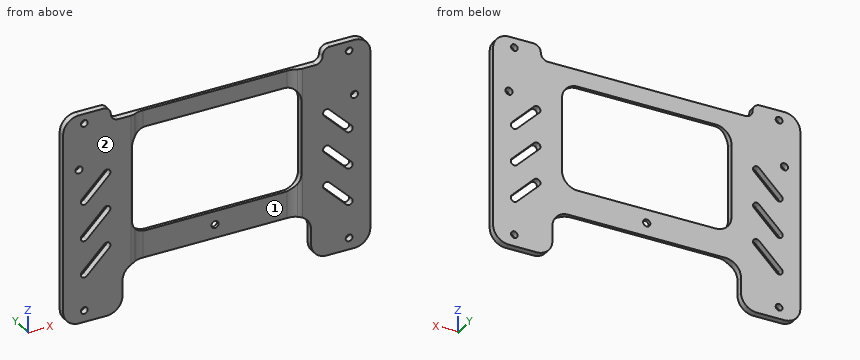
from build123d import *

# Parameters (mm, degrees)
SKETCH_1_R          = 1.7
EXTRUDE_1_DEPTH     = 3
FILLET_1_R          = 7.5
FILLET_2_R          = 3.5
CUT_EXTRUDE_5_DEPTH = 10
CUT_EXTRUDE_6_DEPTH = 10
CUT_EXTRUDE_7_DEPTH = 1.5
FILLET_START        = -35.28
FILLET_3_DEPTH      = 78.28
FILLET_4_R          = 10


with BuildPart() as part:
    # 草图1 → 凸台-拉伸1 (new body)
    with BuildSketch(Plane(origin=(0, 0, 0), x_dir=(1, 0, 0), z_dir=(0, 1, 0))):
        Polygon((-67.5, 50), (-44.5, 50), (-44.5, 27.78), (44.5, 27.78), (44.5, 50), (67.5, 50), (72.5, 50), (72.5, -50), (67.5, -50), (50, -50), (50, -43), (0, -43), (-50, -43), (-50, -50), (-67.5, -50), (-72.5, -50), (-72.5, 50), align=None)
        with Locations(Location((0, 21.39, 0), (0, 0, 270))):
            Circle(SKETCH_1_R, mode=Mode.SUBTRACT)
        with Locations(Location((65, -23.76, 0), (0, 0, 270))):
            Circle(SKETCH_1_R, mode=Mode.SUBTRACT)
        with Locations(Location((-65, -23.76, 0), (0, 0, 270))):
            Circle(SKETCH_1_R, mode=Mode.SUBTRACT)
        Polygon((-40, -10), (-40, -35), (40, -35), (40, 15), (-40, 15), align=None, mode=Mode.SUBTRACT)
    extrude(amount=EXTRUDE_1_DEPTH)

    # 圆角1
    fillet_1_edges = [part.edges().sort_by_distance(p)[0] for p in [
        (72.5, 1.5, -50),
        (72.5, 1.5, 50),
        (-72.5, 1.5, 50),
        (-72.5, 1.5, -50),
        (-44.5, 1.5, -50),
        (-44.5, 1.5, -27.78),
        (44.5, 1.5, -27.78),
        (44.5, 1.5, -50),
        (-40, 1.5, -15),
        (-40, 1.5, 35),
        (40, 1.5, 35),
        (40, 1.5, -15),
    ]]
    fillet(fillet_1_edges, radius=FILLET_1_R)

    # 圆角2
    fillet_2_edges = [part.edges().sort_by_distance(p)[0] for p in [
        (50, 1.5, 43),
        (-50, 1.5, 43),
    ]]
    fillet(fillet_2_edges, radius=FILLET_2_R)
    fillet_2_2_edges = [part.edges().sort_by_distance(p)[0] for p in [
        (50, 1.5, 50),
        (-50, 1.5, 50),
    ]]
    fillet(fillet_2_2_edges, radius=FILLET_2_R - 0.0001)  # a hair under: the kernel refuses the full size

    # 草图12 → 切除-拉伸5 (cut)
    with BuildSketch(Plane(origin=(0, 0, 0), x_dir=(-1, 0, 0), z_dir=(0, -1, 0))):
        with BuildLine():
            ThreePointArc((62.47765, -43.808317961), (61.34627915, -44.276947111), (60.87765, -45.408317961))
            Line((60.87765, -45.408317961), (62.47765, -45.408317961))
            Line((62.47765, -45.408317961), (62.47765, -43.808317961))
        make_face()
        with BuildLine():
            Line((62.47765, -45.408317961), (60.87765, -45.408317961))
            ThreePointArc((60.87765, -45.408317961), (62.47765, -47.008317961), (64.07765, -45.408317961))
            ThreePointArc((64.07765, -45.408317961), (63.60902085, -44.276947111), (62.47765, -43.808317961))
            Line((62.47765, -43.808317961), (62.47765, -45.408317961))
        make_face()
        with BuildLine():
            ThreePointArc((-62.47765, -43.808317961), (-63.60902085, -46.539688811), (-60.87765, -45.408317961))
            Line((-60.87765, -45.408317961), (-62.47765, -45.408317961))
            Line((-62.47765, -45.408317961), (-62.47765, -43.808317961))
        make_face()
        with BuildLine():
            Line((-62.47765, -45.408317961), (-60.87765, -45.408317961))
            ThreePointArc((-60.87765, -45.408317961), (-61.34627915, -44.276947111), (-62.47765, -43.808317961))
            Line((-62.47765, -43.808317961), (-62.47765, -45.408317961))
        make_face()
        with BuildLine():
            ThreePointArc((-62.47765, 42.891807039), (-61.34627915, 43.360436189), (-60.87765, 44.491807039))
            Line((-60.87765, 44.491807039), (-62.47765, 44.491807039))
            Line((-62.47765, 44.491807039), (-62.47765, 42.891807039))
        make_face()
        with BuildLine():
            Line((-62.47765, 44.491807039), (-60.87765, 44.491807039))
            ThreePointArc((-60.87765, 44.491807039), (-63.60902085, 45.623177889), (-62.47765, 42.891807039))
            Line((-62.47765, 42.891807039), (-62.47765, 44.491807039))
        make_face()
        with BuildLine():
            ThreePointArc((64.07765, 44.491807039), (62.47765, 46.091807039), (60.87765, 44.491807039))
            Line((60.87765, 44.491807039), (62.47765, 44.491807039))
            Line((62.47765, 44.491807039), (62.47765, 42.891807039))
            ThreePointArc((62.47765, 42.891807039), (63.60902085, 43.360436189), (64.07765, 44.491807039))
        make_face()
        with BuildLine():
            Line((62.47765, 44.491807039), (60.87765, 44.491807039))
            ThreePointArc((60.87765, 44.491807039), (61.34627915, 43.360436189), (62.47765, 42.891807039))
            Line((62.47765, 42.891807039), (62.47765, 44.491807039))
        make_face()
    extrude(amount=-CUT_EXTRUDE_5_DEPTH, mode=Mode.SUBTRACT)

    # 草图13 → 切除-拉伸6 (cut)
    with BuildSketch(Plane(origin=(0, 3, 0), x_dir=(1, 0, 0), z_dir=(0, 1, 0))):
        with BuildLine():
            Line((61.275568472, -6.806111433), (50.668966754, -17.412713151))
            ThreePointArc((50.668966754, -17.412713151), (50.668966754, -19.816876207), (53.07312981, -19.816876207))
            Line((53.07312981, -19.816876207), (63.679731528, -9.210274489))
            ThreePointArc((63.679731528, -9.210274489), (63.679731528, -6.806111433), (61.275568472, -6.806111433))
        make_face()
        with BuildLine():
            Line((-61.275568472, 28.193888567), (-50.668966754, 17.587286849))
            ThreePointArc((-50.668966754, 17.587286849), (-50.668966754, 15.183123793), (-53.07312981, 15.183123793))
            Line((-53.07312981, 15.183123793), (-63.679731528, 25.789725511))
            ThreePointArc((-63.679731528, 25.789725511), (-63.679731528, 28.193888567), (-61.275568472, 28.193888567))
        make_face()
        with BuildLine():
            Line((-63.679731528, 8.289725511), (-53.07312981, -2.316876207))
            ThreePointArc((-53.07312981, -2.316876207), (-50.668966754, -2.316876207), (-50.668966754, 0.087286849))
            Line((-50.668966754, 0.087286849), (-61.275568472, 10.693888567))
            ThreePointArc((-61.275568472, 10.693888567), (-63.679731528, 10.693888567), (-63.679731528, 8.289725511))
        make_face()
        with BuildLine():
            Line((-63.679731528, -9.210274489), (-53.07312981, -19.816876207))
            ThreePointArc((-53.07312981, -19.816876207), (-50.668966754, -19.816876207), (-50.668966754, -17.412713151))
            Line((-50.668966754, -17.412713151), (-61.275568472, -6.806111433))
            ThreePointArc((-61.275568472, -6.806111433), (-63.679731528, -6.806111433), (-63.679731528, -9.210274489))
        make_face()
        with BuildLine():
            Line((61.275568472, 10.693888567), (50.668966754, 0.087286849))
            ThreePointArc((50.668966754, 0.087286849), (50.668966754, -2.316876207), (53.07312981, -2.316876207))
            Line((53.07312981, -2.316876207), (63.679731528, 8.289725511))
            ThreePointArc((63.679731528, 8.289725511), (63.679731528, 10.693888567), (61.275568472, 10.693888567))
        make_face()
        with BuildLine():
            Line((61.275568472, 28.193888567), (50.668966754, 17.587286849))
            ThreePointArc((50.668966754, 17.587286849), (50.668966754, 15.183123793), (53.07312981, 15.183123793))
            Line((53.07312981, 15.183123793), (63.679731528, 25.789725511))
            ThreePointArc((63.679731528, 25.789725511), (63.679731528, 28.193888567), (61.275568472, 28.193888567))
        make_face()
    extrude(amount=-CUT_EXTRUDE_6_DEPTH, mode=Mode.SUBTRACT)

    # 草图14 → 切除-拉伸7 (cut)
    with BuildSketch(Plane.XZ):
        Polygon((-37, 27.78), (-37, 43), (37, 43), (37, 27.78), (37, -27.78), (-37, -27.78), align=None)
    extrude(amount=-CUT_EXTRUDE_7_DEPTH, mode=Mode.SUBTRACT)

    # 圆角3: read off the stored shape, not the designer's step
    # 圆角3 outline → 圆角3 (cut)
    with BuildSketch(Plane.XY.offset(FILLET_START)):
        with BuildLine():
            Line((-40.570714214, 0), (-37, 0))
            Line((-37, 0), (-37, 1.5))
            ThreePointArc((-37, 1.5), (-38.634222541, 0.390227771), (-40.570714214, 0))
        make_face()
        with BuildLine():
            ThreePointArc((40.570714214, 0), (38.634222541, 0.390227771), (37, 1.5))
            Line((37, 1.5), (37, 0))
            Line((37, 0), (40.570714214, 0))
        make_face()
    extrude(amount=FILLET_3_DEPTH, mode=Mode.SUBTRACT)

    # 圆角4
    fillet_4_edges = [part.edges().sort_by_distance(p)[0] for p in [
        (-37, 1.5, 38.25),
        (-37, 1.5, -20.64),
        (37, 1.5, 38.25),
        (37, 1.5, -20.64),
    ]]
    fillet(fillet_4_edges, radius=FILLET_4_R)


solid = part.part
Input: part model. Units: mm. Frame: model coordinates. Face numbers are marked on the shaded views. Coordinates: 2 decimals unless noted, no trailing zeros. Write each loop counter-clockwise with the first axis right and the second up, starting at its lowest first coordinate (ties: lowest second). Pieces come first, ordered by that corner, then holes. Notation, with made-up numbers: M 35.25,29 L 89.25,29 A21 cw 89.25,67 Z; hole C 11,15.5 d7. An arc over 180 degrees is marked long. Answer as a JSON object with one key per item and string values. Group by question number.
(1) Ray query, line 1 along Z through (x, y) = (0, 2.6); line 2 along X through (y, z) = (1.75, 23.76); line 3 along Z through (x, y) = (65, 1.75). Return the intervals inside material, ascending. Write a range as [from, to].
(2) Section A-A on z = 23.76. Output: boundary loops of the cut face in (x, y), plus the area to 3 significant figures.
(3) Section B-B on x = -20. Output: boundary loops of the cut face in (y, z), plus the area to 3 significant figures.
(4) Section C-C on x = 0. Output: boundary loops of the cut face in (y, z), plus the area to 3 significant figures.
(5) Section D-D on z = 37. Output: boundary loops of the cut face in (x, y).
(6) Mould query, pull axis X, two halves, no side actions, for the marked faces 1 and 2. Classes: pulls with the +X half, pulls with the -X half, needs draft (parallel to the pull), parting line crosses it, or undercut.
(7) Contact query for flat-ended pins moving along their axis: P1, Ø1, axis at x = 50, y = 2, coming from the -Z side; P2, Ø1.2, axis at x = -11.5, y = 2, coming from the -Z side; P3, Ø6.5, axis at x = -9.5, z = -21.5, coming from the -Y side; P4, Ø2.5, axis at x = 65, z = 23.76, coming from the +Y side. Output: stop coordinate, or through.
Result set:
{
 "1": {"line 1": "z = [-27.78, -23.09], [-19.69, -15], [35, 43]", "line 2": "x = [-72.5, -66.7], [-63.3, -40], [40, 63.3], [66.7, 72.5]", "line 3": "z = [-50, 22.06], [25.46, 50]"},
 "2": {"outline": "M -72.5,0 L -66.7,0 L -66.7,3 L -72.5,3 Z; M -63.3,0 L -40.57,0 A5 ccw -40,0.03 L -40,3 L -63.3,3 Z; M 40,0.03 A5 ccw 40.57,0 L 63.3,0 L 63.3,3 L 40,3 Z; M 66.7,0 L 72.5,0 L 72.5,3 L 66.7,3 Z", "area": "175 mm2"},
 "3": {"outline": "M 1.5,-27.78 L 3,-27.78 L 3,-15 L 1.5,-15 Z; M 1.5,35 L 3,35 L 3,43 L 1.5,43 Z", "area": "31.2 mm2"},
 "4": {"outline": "M 1.5,-27.78 L 3,-27.78 L 3,-23.09 L 1.5,-23.09 Z; M 1.5,-19.69 L 3,-19.69 L 3,-15 L 1.5,-15 Z; M 1.5,35 L 3,35 L 3,43 L 1.5,43 Z", "area": "26.1 mm2"},
 "5": {"outline": "M -72.5,0 L -40.57,0 A5 ccw -38.39,0.5 A10 cw -34.03,1.5 L 34.03,1.5 A10 cw 38.39,0.5 A5 ccw 40.57,0 L 72.5,0 L 72.5,3 L -72.5,3 Z"},
 "6": {"face 1": "undercut", "face 2": "needs draft"},
 "7": {"P1": "stops at z = -49.85", "P2": "stops at z = -27.78", "P3": "stops at y = 1.5", "P4": "passes through"}
}
